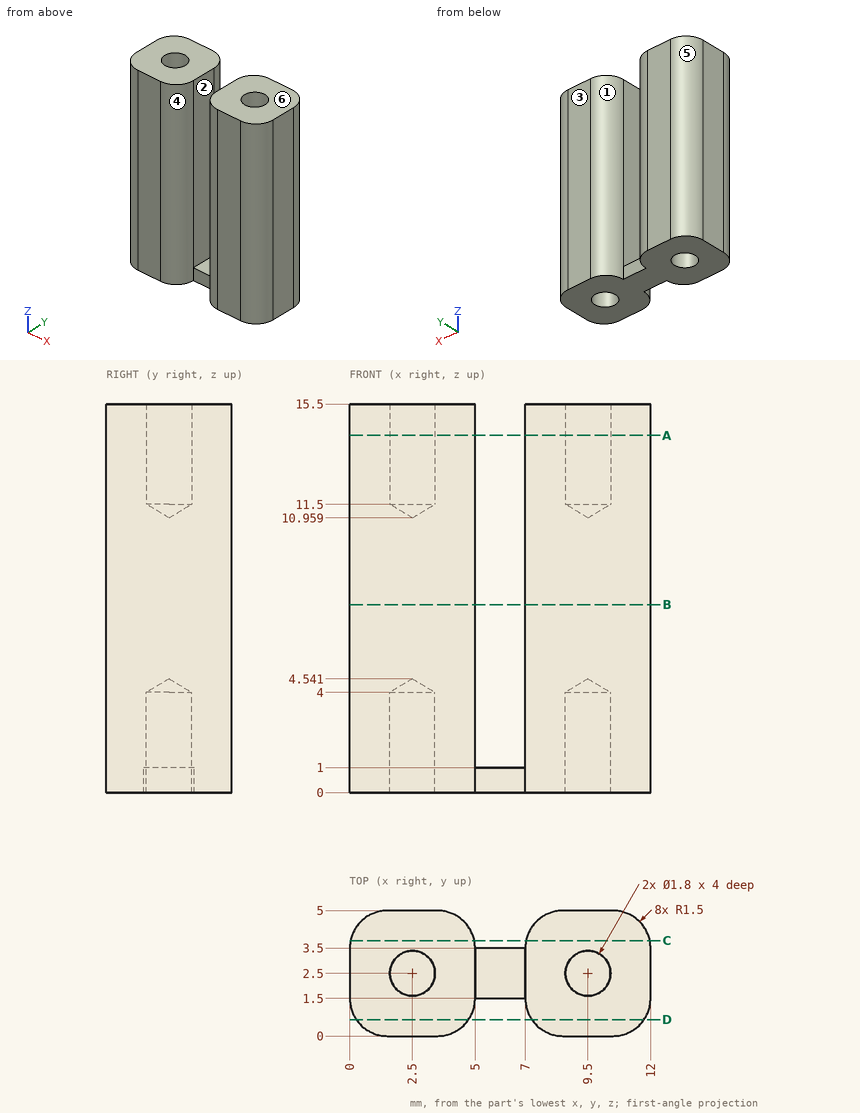
Geometry: see drawing. Coordinates: mm, zero at the bounding-box minimum. A direction names the side the tool comes from. Coordinates: 2 decimals unless noted, no trailing zeros. Write each loop counter-clockwise with the first axis right and the second up, starting at its lowest first coordinate (ties: lowest second). Pieces come first, ordered by that corner, then holes. Notation, with made-up numbers: M 58.5,24 L 94.5,24 A16 ccw 94.5,41 Z; hole C 46,82.5 d5. An arc over 180 degrees is marked long. Answer as a JSON object with one key per item and string values.
1. Cut plane C-C on y = 3.8. Output: boundary loops of the cut face in (x, z), plus the area to 3 significant figures.
Evaluation:
{"outline": "M 0.03,0 L 4.97,0 L 4.97,15.5 L 0.03,15.5 Z; M 7.03,0 L 11.97,0 L 11.97,15.5 L 7.03,15.5 Z", "area": "153 mm^2"}
2. Contact query for flat-ended pins moving along their axis: P1, Ø0.5, axis at x = 6, z = 0.5, coming from the +Y side; P2, Ø1.5, axis at x = 7.5, z = 9, coming from the -Y side; P3, Ø1, axis at y = 0.5, z = 2, coming from the -X side. Output: stop coordinate, or through.
Evaluation:
{"P1": "y = 3.5", "P2": "y = 0.02", "P3": "x = 0.09"}
3. Cut plane D-D on y = 0.65. Output: boundary loops of the cut face in (x, z).
Evaluation:
{"outline": "M 0.26,0 L 4.74,0 L 4.74,15.5 L 0.26,15.5 Z; M 7.26,0 L 11.74,0 L 11.74,15.5 L 7.26,15.5 Z"}
4. Cut plane B-B on z = 7.5. Output: boundary loops of the cut face in (x, y).
Evaluation:
{"outline": "M 0,1.5 A1.5 ccw 1.5,0 L 3.5,0 A1.5 ccw 5,1.5 L 5,3.5 A1.5 ccw 3.5,5 L 1.5,5 A1.5 ccw 0,3.5 Z; M 7,1.5 A1.5 ccw 8.5,0 L 10.5,0 A1.5 ccw 12,1.5 L 12,3.5 A1.5 ccw 10.5,5 L 8.5,5 A1.5 ccw 7,3.5 Z"}
5. Draft query along X for the marked faces 4, 5 and 6. Return one class per face: released by +X, released by -X, zero draft, split by the parting line, or undercut.
Evaluation:
{"face 4": "undercut", "face 5": "released by -X", "face 6": "zero draft"}
6. Cut plane A-A on z = 14.25. Output: boundary loops of the cut face in (x, y).
Evaluation:
{"outline": "M 0,1.5 A1.5 ccw 1.5,0 L 3.5,0 A1.5 ccw 5,1.5 L 5,3.5 A1.5 ccw 3.5,5 L 1.5,5 A1.5 ccw 0,3.5 Z; M 7,1.5 A1.5 ccw 8.5,0 L 10.5,0 A1.5 ccw 12,1.5 L 12,3.5 A1.5 ccw 10.5,5 L 8.5,5 A1.5 ccw 7,3.5 Z; hole C 2.5,2.5 d1.8; hole C 9.5,2.5 d1.8"}
7. Access query for the marked faces 1, 2 and 3. Directions: +Z, -Z, +X, -X, +Y, -Y. A direction counts if a zero-diameter tool reaches every point of the face in a straight line with its end or side. Return the directions, or none.
Evaluation:
{"face 1": "+Z, -Z, +Y", "face 2": "+Z, +Y, -Y", "face 3": "+Z, -Z, +X, -X, +Y"}
8. Ray query, L1, parallel to X at y = 3.2, z = 9.75; L2, parallel to Y at x = 9.5, z = 2.65; L3, parallel to X at y = 3.05, z = 11.75. Return the intervals inside material, ascending.
Evaluation:
{"L1": "0 to 5, 7 to 12", "L2": "0 to 1.6, 3.4 to 5", "L3": "0 to 1.79, 3.21 to 5, 7 to 8.79, 10.21 to 12"}
